Read the model definition and answer for the solid it produces. Units are mm, in the model's axes. A direction names the side the tool comes from. Coordinates: 2 decimals unless noted, no trailing zeros. Loops run counter-clockwise (first coordinate to the right, second up) from the corner with the lowest first, then second, coordinate; pieces in that order, holes last. Notation, with made-up numbers: (13, 60) - (68, 60) arc R26 cw to (68, 85) - close; hole circle Ø9 at (53, 74.25). An arc over 180 degrees is marked (long way). Use one line per item in the form item = value. Start each with the question number.
1) Which of the six approach directions +Z, -Z, +X, -X, +Y, -Y give full straight-line access (tool end or side, diameter ignored) to faces 4 (the face through (25, -41, 40)), 5 (the face through (-41.281, 29.648, 15.768))?
2) Each of these flat-tipped pins is pushed along its axis until it touches: P1, Ø7, axis at x = 41.76, y = -27.5, coming from the +Z side; P2, Ø8, axis at x = 27.5, y = 41.76, coming from the -Z side; P3, Ø6, axis at x = 37.5, z = 33, coming from the +Y side. Where does it stop, or does it pass through?
3) A cutting plane is placed at C-C (y = 15). Give the vertices of the cut face in (x, z), and give its area (3 significant figures).
4) The mould has two halves that part along X. Classify faces 1 (the face through (-40.63, -44.15, 16.23)), 2 (the face through (0, 50, 21)), 3 (the face through (31.673, -43.072, 19.72)): released by +X, released by -X, zero draft, split by the parting line, or undercut.
5) Consider line 1 (Y direction, x = -27, z = 19); line 2 (Y direction, x = 24, z = 14); line 3 (Y direction, x = -16.5, z = 39). Determine where each line is inside the solid, lowest interval first.
6) A cutting plane is placed at A-A (y = -27.5). Give the vertices of the cut face in (x, z).
7) A cutting plane is placed at B-B (x = 18.5). Give the vertices of the cut face in (y, z), and give its area (3 significant figures).
8) A cutting plane is placed at D-D (x = 7.5). Give the vertices of the cut face in (y, z), and give its area (3 significant figures).
from build123d import *

# Parameters (mm, degrees)
F1_DEPTH         = 42.5
F3_DEPTH         = 25.5
F4_R             = 12.5
F5_DEPTH         = 100.001
F6_R             = 12.5
F7_DEPTH         = 100.0010000004
F9_D             = 4.4
F9_CBORE_D       = 8.75
F9_CBORE_DEPTH   = 40
F10_D            = 4.4
F11_R            = 2.2
F12_DEPTH        = 14.5
F15_D            = 2
F15_DEPTH        = 7.5
F15_TIP          = 0.600860619
F15_ON_F13_D     = 2
F15_ON_F13_DEPTH = 7.5
F15_ON_F13_TIP   = 0.600860619


with BuildPart() as f1:
    # F0 (on Top) → F1 (new body)
    with BuildSketch(Plane.XY):
        with BuildLine():
            Line((33.1662479036, 50), (-33.1662479036, 50))
            ThreePointArc((-33.1662479036, 50), (-42.4264068712, 42.4264068712), (-50, 33.1662479036))
            Line((-50, 33.1662479036), (-50, -33.1662479036))
            ThreePointArc((-50, -33.1662479036), (-42.4264068712, -42.4264068712), (-33.1662479036, -50))
            Line((-33.1662479036, -50), (33.1662479036, -50))
            ThreePointArc((33.1662479036, -50), (42.4264068712, -42.4264068712), (50, -33.1662479036))
            Line((50, -33.1662479036), (50, 33.1662479036))
            ThreePointArc((50, 33.1662479036), (42.4264068712, 42.4264068712), (33.1662479036, 50))
        make_face()
    extrude(amount=F1_DEPTH)

    # F2 (on face) → F3 (cut)
    with BuildSketch(Plane.XY.offset(42.5)):
        with BuildLine():
            Line((-29.8585786438, 30), (-42.3556372675, 42.4970586237))
            ThreePointArc((-42.3556372675, 42.4970586237), (-42.3910367885, 42.4617474911), (-42.4264068712, 42.4264068712))
            ThreePointArc((-42.4264068712, 42.4264068712), (-46.4445670429, 37.985552414), (-50, 33.1662479036))
            Line((-50, 33.1662479036), (-50, -33.1662479036))
            ThreePointArc((-50, -33.1662479036), (-46.4128962783, -38.0242430438), (-42.3556372675, -42.4970586237))
            Line((-42.3556372675, -42.4970586237), (-29.8585786438, -30))
            Line((-29.8585786438, -30), (29.8585786438, -30))
            Line((29.8585786438, -30), (42.3556372675, -42.4970586237))
            ThreePointArc((42.3556372675, -42.4970586237), (42.3910367885, -42.4617474911), (42.4264068712, -42.4264068712))
            ThreePointArc((42.4264068712, -42.4264068712), (46.4445670429, -37.985552414), (50, -33.1662479036))
            Line((50, -33.1662479036), (50, 33.1662479036))
            ThreePointArc((50, 33.1662479036), (46.4445670429, 37.985552414), (42.4264068712, 42.4264068712))
            ThreePointArc((42.4264068712, 42.4264068712), (42.3910367885, 42.4617474911), (42.3556372675, 42.4970586237))
            Line((42.3556372675, 42.4970586237), (29.8585786438, 30))
            Line((29.8585786438, 30), (-29.8585786438, 30))
        make_face()
    extrude(amount=-F3_DEPTH, mode=Mode.SUBTRACT)

    # F4 (on face) → F5 (cut, through all)
    with BuildSketch(Plane.XZ.offset(50)):
        with Locations((0, 43)):
            Circle(F4_R)
    extrude(amount=-F5_DEPTH, mode=Mode.SUBTRACT)

    # F6 (on face) → F7 (cut, through all)
    with BuildSketch(Plane.YZ.offset(50)):
        with Locations((0, 17.5)):
            Circle(F6_R)
    extrude(amount=-F7_DEPTH, mode=Mode.SUBTRACT)

    # F9 (through all)
    with Locations(Plane(origin=(0, 0, 0), x_dir=(1, 0, 0), z_dir=(0, 0, -1))):
        with Locations((-27.5, 41.7582327212), (27.5, 41.7582327212), (27.5, -41.7582327212), (-27.5, -41.7582327212)):
            CounterBoreHole(F9_D / 2, F9_CBORE_D / 2, F9_CBORE_DEPTH)

    # F10 (through all)
    with Locations(Plane(origin=(0, 0, 0), x_dir=(1, 0, 0), z_dir=(0, 0, -1))):
        with Locations((-41.7582327212, 27.5), (-41.7582327212, -27.5), (41.7582327212, -27.5), (41.7582327212, 27.5)):
            Hole(F10_D / 2)

    # F11 (on face) → F12 (cut)
    with BuildSketch(Plane(origin=(0, 0, 0), x_dir=(1, 0, 0), z_dir=(0, 0, -1))):
        Polygon((-41.7582327212, 23.1698729811), (-38.0082327212, 25.3349364905), (-38.0082327212, 29.6650635095), (-41.7582327212, 31.8301270189), (-45.5082327212, 29.6650635095), (-45.5082327212, 25.3349364905), align=None)
        with Locations((-41.7582327212, 27.5)):
            Circle(F11_R, mode=Mode.SUBTRACT)
        Polygon((38.0082327212, 29.6650635095), (38.0082327212, 25.3349364905), (41.7582327212, 23.1698729811), (45.5082327212, 25.3349364905), (45.5082327212, 29.6650635095), (41.7582327212, 31.8301270189), align=None)
        with Locations((41.7582327212, 27.5)):
            Circle(F11_R, mode=Mode.SUBTRACT)
        Polygon((41.7582327212, -23.1698729811), (38.0082327212, -25.3349364905), (38.0082327212, -29.6650635095), (41.7582327212, -31.8301270189), (45.5082327212, -29.6650635095), (45.5082327212, -25.3349364905), align=None)
        with Locations((41.7582327212, -27.5)):
            Circle(F11_R, mode=Mode.SUBTRACT)
        Polygon((-41.7582327212, -31.8301270189), (-38.0082327212, -29.6650635095), (-38.0082327212, -25.3349364905), (-41.7582327212, -23.1698729811), (-45.5082327212, -25.3349364905), (-45.5082327212, -29.6650635095), align=None)
        with Locations((-41.7582327212, -27.5)):
            Circle(F11_R, mode=Mode.SUBTRACT)
    extrude(amount=-F12_DEPTH, mode=Mode.SUBTRACT)

    # F15
    with Locations(Plane(origin=(0, 0, 0), x_dir=(1, 0, 0), z_dir=(0, 0, -1))):
        with Locations((-30, 30), (30, 30), (30, -30), (-30, -30)):
            Hole(F15_D / 2, depth=F15_DEPTH)
            with Locations((0, 0, -(F15_DEPTH + F15_TIP / 2))):  # 118° drill point
                Cone(0, F15_D / 2, F15_TIP, mode=Mode.SUBTRACT)

    # F15 on F13
    with Locations(Plane(origin=(0, 0, 0), x_dir=(1, 0, 0), z_dir=(0, 0, -1))):
        with Locations((31.8, 8.85), (31.8, -19.05), (-20.3, -24.15), (-19, 24.05)):
            Hole(F15_ON_F13_D / 2, depth=F15_ON_F13_DEPTH)
            with Locations((0, 0, -(F15_ON_F13_DEPTH + F15_ON_F13_TIP / 2))):  # 118° drill point
                Cone(0, F15_ON_F13_D / 2, F15_ON_F13_TIP, mode=Mode.SUBTRACT)


solid = f1.part
Found:
q1.face_4 = -Z
q1.face_5 = +Z, -Z
q2.P1 = 17
q2.P2 = 40
q2.P3 = 49.09
q3.outline = (-50, 0) - (50, 0) - (50, 17) - (-50, 17) - close
q3.area = 1,700 mm^2
q4.face_1 = released by -X
q4.face_2 = zero draft
q4.face_3 = undercut
q5.line_1 = -50 to -46.1, -37.41 to -30, 30 to 37.41, 46.1 to 50
q5.line_2 = -50 to -44.38, -39.13 to -12, 12 to 39.13, 44.38 to 50
q5.line_3 = -50 to -30, 30 to 50
q6.outline = (-50, 0) - (-45.51, 0) - (-45.51, 14.5) - (-43.96, 14.5) - (-43.96, 17) - (-50, 17) - close; (-39.56, 14.5) - (-38.01, 14.5) - (-38.01, 0) - (38.01, 0) - (38.01, 14.5) - (39.56, 14.5) - (39.56, 17) - (-39.56, 17) - close; (43.96, 14.5) - (45.51, 14.5) - (45.51, 0) - (50, 0) - (50, 17) - (43.96, 17) - close
q7.outline = (-50, 0) - (50, 0) - (50, 42.5) - (30, 42.5) - (30, 17) - (12.49, 17) arc R12.5 cw to (-12.49, 17) - (-30, 17) - (-30, 42.5) - (-50, 42.5) - close
q7.area = 2,490 mm^2
q8.outline = (-50, 0) - (50, 0) - (50, 33) - (30, 33) - (30, 17) - (12.49, 17) arc R12.5 cw to (-12.49, 17) - (-30, 17) - (-30, 33) - (-50, 33) - close
q8.area = 2,110 mm^2
